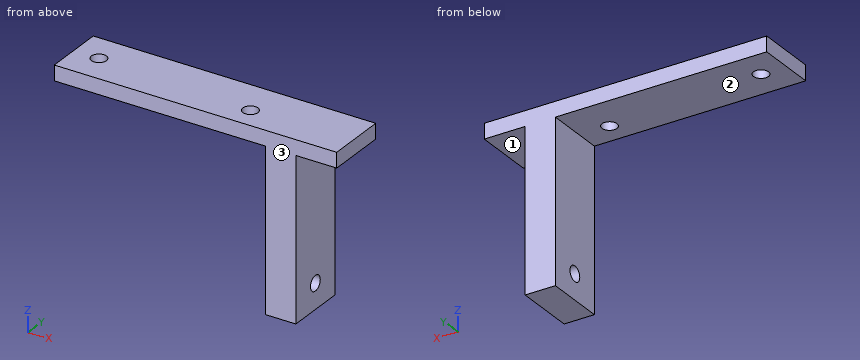
Autodesk Inventor part; units mm, degrees
ref_plane "YZ Plane" through (0, 0, 0) normal (1, 0, 0) x (0, 1, 0)
ref_plane "XZ Plane" through (0, 0, 0) normal (0, 1, 0) x (-1, 0, 0)
ref_plane "XY Plane" through (0, 0, 0) normal (0, 0, 1) x (1, 0, 0)
sketch "Sketch3" plane through (0, 0, 0) normal (0, 0, 1) x (1, 0, 0)
  line L0 (0, 0) -> (56, 0)
  line L1 (56, 0) -> (56, 12)
  line L2 (56, 12) -> (0, 12)
  line L3 (0, 12) -> (0, 0)
  circle A0 centre (36, 4.5) radius 1.5
  circle A1 centre (5, 6) radius 1.5
  dimension "d0" = 56
  dimension "d2" = 3
  dimension "d3" = 4.5
  dimension "d4" = 12
  dimension "d8" = 20
  dimension "d17" = 3
  dimension "d18" = 5
extrude "Extrusion1" add sketch "Sketch3" along normal blind 3
sketch "Sketch4" plane through (0, 0, 3) normal (0, 0, 1) x (1, 0, 0)
  line L0 (56, 12) -> (0, 12)
  line L1 (41.9, 0) -> (47.9, 0)
  line L2 (47.9, 0) -> (47.9, 12)
  line L3 (47.9, 12) -> (41.9, 12)
  line L4 (41.9, 12) -> (41.9, 0)
  circle A0 centre (36, 4.5) radius 1.5
  point P0 (0, 0)
  dimension "d9" = 6
  dimension "d10" = 5.9
extrude "Extrusion2" add sketch "Sketch4" against normal blind 35 contours L2 L1 L4 L0
sketch "Sketch5" plane through (47.9, 0, 0) normal (1, 0, 0) x (0, 0, -1)
  line L0 (32, 0) -> (32, 12) construction
  line L1 (0, 6) -> (0, 3) construction
  line L2 (32, 6) -> (0, 6) construction
  circle A0 centre (27, 6) radius 1.5
  point P0 (0, 0)
  dimension "d13" = 3
  dimension "d14" = 5
extrude "Extrusion3" cut sketch "Sketch5" against normal through all
properties part number "thumper-bumper-solenoid-interface-v2"
Check sheet for the modelled part. Datum: model origin and axes. Units: mm. Face numbers are marked on the shaded views. A direction names the side the tool comes from. Round coordinates to 2 decimals unless told otherwise and drop trailing zeros. Loops run counter-clockwise (first coordinate to the right, second up) from the corner with the lowest first, then second, coordinate; pieces in that order, holes last. Notation, with made-up numbers: M 30,81.5 L 38,81.5 A20 ccw 38,98.5 Z; hole C -26.75,8 d9. An arc over 180 degrees is marked long. One line per question, with ' | ' between items. Start each with the question number.
Item 1: Gauge pin test, flat ends, axial feed: pin 1 Ø4 at (x, y) = (36, 4.5) entering from -Z; pin 2 Ø2.5 at (y, z) = (6, -27) entering from +X (3 decimals). Record the tip position at first contact, or that the pin passes through.
Item 2: Scan lines: probe 1 along Y at (x, z) = (5, 1); probe 2 along Z at (x, y) = (20, 8); probe 3 along X at (y, z) = (9.5, -28). Record each from-to range of solid material in increasing order.
Item 3: Section check D-D (z = -19). Record the boundary of the cut face in (x, y), and give its area (3 significant figures).
Item 4: Section check B-B (z = -27). Record the boundary of the cut face in (x, y).
Item 5: Section check C-C (y = 8.5). Record the boundary of the cut face in (x, z).
Item 6: Section check A-A (x = 5). Record the boundary of the cut face in (y, z).
Item 7: Set-up check for the marked faces 1, 2 and 3: record each of +Z, -Z, +X, -X, +Y, -Y from which the full face is reachable in a straight line by a thin tool's end or side.
Worked out:
1) pin 1: z = 0 | pin 2: through
2) probe 1: 0 to 4.5, 7.5 to 12 | probe 2: 0 to 3 | probe 3: 41.9 to 47.9
3) outline: M 41.9,0 L 47.9,0 L 47.9,12 L 41.9,12 Z | area: 72.0 mm^2
4) outline: M 41.9,0 L 47.9,0 L 47.9,4.5 L 41.9,4.5 Z; M 41.9,7.5 L 47.9,7.5 L 47.9,12 L 41.9,12 Z
5) outline: M 0,0 L 41.9,0 L 41.9,-32 L 47.9,-32 L 47.9,0 L 56,0 L 56,3 L 0,3 Z
6) outline: M 0,0 L 4.5,0 L 4.5,3 L 0,3 Z; M 7.5,0 L 12,0 L 12,3 L 7.5,3 Z
7) face 1: -Z, +X, +Y, -Y | face 2: -Z, -X, +Y, -Y | face 3: +Z, -Z, +X, -X, -Y
